Build history of the part. All positions in model axes, mm. Face numbers are marked on the shaded views. A direction names the side the tool comes from. Round coordinates to 2 decimals unless told otherwise and drop trailing zeros. Write each loop counter-clockwise with the first axis right and the second up, starting at its lowest first coordinate (ties: lowest second). Pieces come first, ordered by that corner, then holes. Notation, with made-up numbers: (34, 75.25) - (61, 75.25) arc R27 ccw to (61, 105.25) - close; hole circle Ø7 at (86, -12.75). An arc over 180 degrees is marked (long way). One line per question, with ' | ' between items.
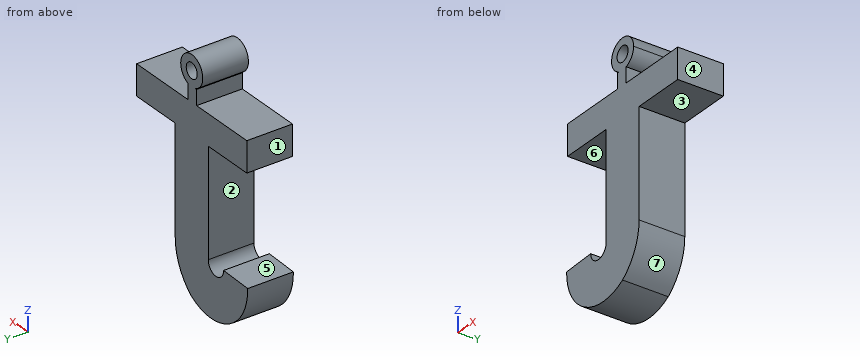
from build123d import *

# Parameters (mm, degrees)
F0_R     = 1.27
F1_DEPTH = 7.62


with BuildPart() as f1:
    # F0 (on Front) → F1 (new body)
    with BuildSketch(Plane.XZ):
        with BuildLine():
            Line((-1.1249838863, 0), (0, 0))
            Line((0, 0), (0.8244126237, 0))
            Line((0.8244126237, 0), (0.8244126237, 2.54))
            ThreePointArc((0.8244126237, 2.54), (0, 2.4024870085), (-0.8244126237, 2.54))
            Line((-0.8244126237, 2.54), (-1.1249838863, 2.54))
            Line((-1.1249838863, 2.54), (-1.1249838863, 0))
        make_face()
        with BuildLine():
            Line((0.8244126237, 0), (0, 0))
            Line((0, 0), (-1.1249838863, 0))
            Line((-1.1249838863, 0), (-12.7, 0))
            Line((-12.7, 0), (-12.7, -5.08))
            Line((-12.7, -5.08), (-3.81, -5.08))
            Line((-3.81, -5.08), (-3.81, -22.86))
            ThreePointArc((-3.81, -22.86), (-5.5788724448, -24.6288724448), (-7.3477448896, -22.86))
            Line((-7.3477448896, -22.86), (-12.896864675, -23.0650249869))
            ThreePointArc((-12.896864675, -23.0650249869), (-8.6576895541, -30.6153855835), (0, -30.4638519883))
            ThreePointArc((0, -30.4638519883), (2.8042172177, -27.1124894197), (3.81, -22.86))
            Line((3.81, -22.86), (3.81, -5.08))
            Line((3.81, -5.08), (12.7, -5.08))
            Line((12.7, -5.08), (12.7, 0))
            Line((12.7, 0), (0.8244126237, 0))
        make_face()
        with BuildLine():
            ThreePointArc((-0.8244126237, 2.54), (0, 2.4024870085), (0.8244126237, 2.54))
            Line((0.8244126237, 2.54), (-0.8244126237, 2.54))
        make_face()
        with BuildLine():
            Line((-0.8244126237, 2.54), (0.8244126237, 2.54))
            ThreePointArc((0.8244126237, 2.54), (2.0670762038, 3.4664124955), (2.54, 4.9424870085))
            ThreePointArc((2.54, 4.9424870085), (-1.476074513, 7.0095632122), (-0.8244126237, 2.54))
        make_face()
        with Locations((0, 4.9424870085)):
            Circle(F0_R, mode=Mode.SUBTRACT)
    extrude(amount=F1_DEPTH)


solid = f1.part
Q1. Saw through at A-A, the plane y = -4.25. List the corners of the cut face in (x, z).
Found:
outline: (-12.9, -23.07) arc R8.44 ccw to (0, -30.46) arc R9.49 ccw to (3.81, -22.86) - (3.81, -5.08) - (12.7, -5.08) - (12.7, 0) - (0.82, 0) - (0.82, 2.54) arc R2.54 ccw (long way) to (-0.82, 2.54) - (-1.12, 2.54) - (-1.12, 0) - (-12.7, 0) - (-12.7, -5.08) - (-3.81, -5.08) - (-3.81, -22.86) arc R1.77 cw to (-7.35, -22.86) - close; hole circle Ø2.54 at (0, 4.94)
Q2. Drill centre lines: L1, parallel to Z at x = 0, y = -4; L2, parallel to X at y = -6.25, z = -12.5; L3, parallel to X at y = -2.25, z = -2. Where is each one in solid material? Low to high. Write a range as from..to.
Found:
L1: -30.46..3.67, 6.21..7.48 | L2: -3.81..3.81 | L3: -12.7..12.7
Q3. Which spindle directions (+Z, -Z, +X, -X, +Y, -Y) get a long thin tool onto all of the face, cutting with end or side? Do the marked faces 1, 2 and 3. Say none if no direction does.
Found:
face 1: +Z, -X, +Y, -Y | face 2: -X, +Y, -Y | face 3: -Z, +X, +Y, -Y
Q4. Drop flat-ended pins along their axis: pin 1 (2 mm diameter, centred on x = -1, y = -6, fed in from -Z); pin 2 (2.5 mm diameter, centred on x = -7.5, y = -3.5, fed in from -Z); pin 3 (3 mm diameter, centred on y = -4.5, z = 2, fed in from +X); pin 4 (10 mm diameter, centred on x = 0.5, z = -11, fed in from +Y). Give the stop position or say it passes through.
Found:
pin 1: z = -31.37 | pin 2: z = -31.54 | pin 3: x = 2.09 | pin 4: y = 0
Q5. Saw through at C-C, the plane x = 9.75. List the corners of the cut face in (y, z).
Found:
outline: (-7.62, -5.08) - (0, -5.08) - (0, 0) - (-7.62, 0) - close
Q6. Saw through at B-B, the plane z = -22. List the corners of the cut face in (x, y), then the cut area to 3 significant figures.
Found:
outline: (-3.81, -7.62) - (3.81, -7.62) - (3.81, 0) - (-3.81, 0) - close | area: 58.1 mm^2
Q7. Pull direction Z, two halves, no side cores. Call the marked faces 4, 5, 6 and 7: +Z half, -Z half, draft (parallel to the pull), parting line (faces both ways), or undercut.
Found:
face 4: draft | face 5: undercut | face 6: undercut | face 7: -Z half
